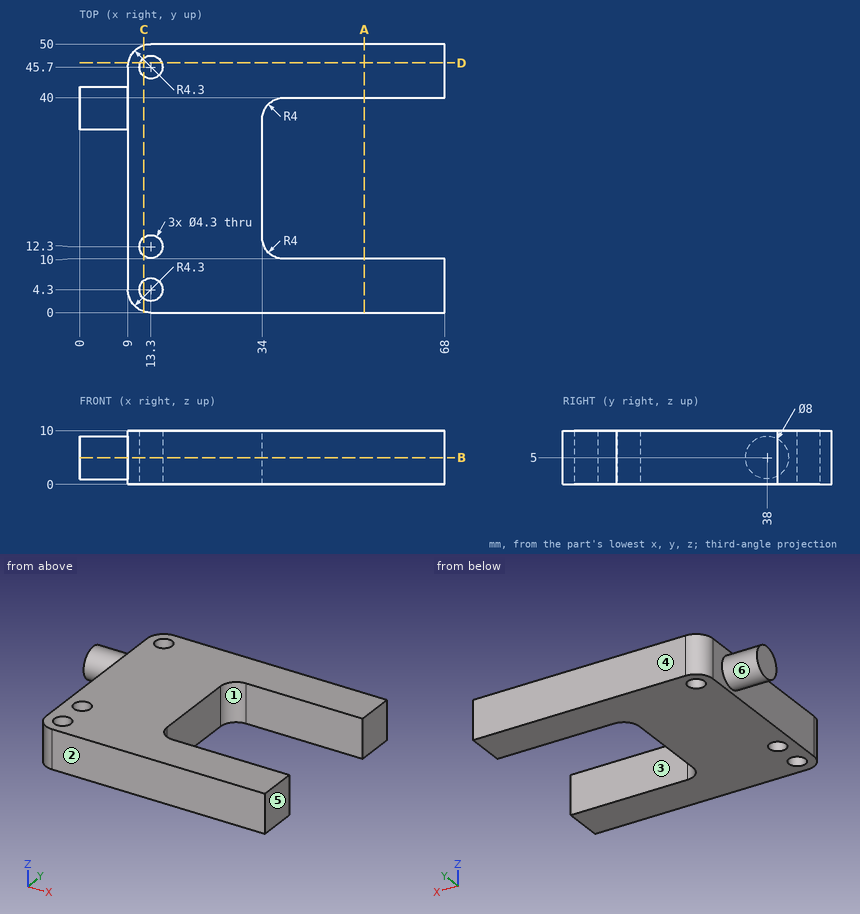
Could you check a few things on this drawing? It's one solid part, dimensions in mm from its lowest x, y, z. A direction names the side the tool comes from. Give positions to 0.01 mm unless a question says otherwise; leave off trailing zeros. Order: outer loops, then holes, each group sorted by start corner. A loop starts at its lowest first (then second) coordinate and runs counter-clockwise, first axis right, second up. Notation, with made-up numbers: (65, -18) - (69, -18) arc R34 cw to (69, 14) - close; hole circle Ø9 at (-2, -27.5). An arc over 180 degrees is marked (long way). One line per question, with ' | ' between items. Start each with the question number.
Item 1: Thinking about a two-plate mould opening in Y: for the marked faces 3, 4, 5 and 6, which applies, pulls with the +Y half, pulls with the -Y half, needs draft (parallel to the pull), parting line crosses it, or undercut?
Item 2: I need wall thicknesses on probe 1 along Y at (x, z) = (13.3, 4.75); probe 2 along Y at (x, z) = (41.5, 1.25); probe 3 along X at (y, z) = (36, 7.5). Which ranges of each line are inside material? Lowest first, please. Write a range as [from, to].
Item 3: I want a section at B-B on z = 5. Write out the boundary of the cut face in (x, y).
Item 4: I want a section at C-C on x = 12. Write out the boundary of the cut face in (y, z).
Item 5: I'm going to push flat-ended pins straight in: pin 1 Ø5 at (y, z) = (19, 5.5) entering from -X; pin 2 Ø5.5 at (x, y) = (13.3, 4.3) entering from -Z; pin 3 Ø1.5 at (y, z) = (37, 6) entering from +X; pin 4 Ø5 at (y, z) = (26, 4) entering from +X. Where does each tip first touch, or does it pass through?
Item 6: For the marked faces 1 and 2, which set-ups out of +Z, -Z, +X, -X, +Y, -Y let a thin tool reach every point of the face, with its end or its side?
Item 7: I want a section at D-D on y = 46.5. Write out the boundary of the cut face in (x, z).
Item 8: I want a section at A-A on x = 53. Write out the boundary of the cut face in (y, z), then the cut area to 3 significant figures.
Verdict:
1) face 3: undercut | face 4: pulls with the +Y half | face 5: needs draft | face 6: parting line crosses it
2) probe 1: [0, 2.15], [6.45, 10.15], [14.45, 43.55], [47.85, 50] | probe 2: [0, 10], [40, 50] | probe 3: [0, 34]
3) outline: (0, 34) - (9, 34) - (9, 4.3) arc R4.3 ccw to (13.3, 0) - (68, 0) - (68, 10) - (38, 10) arc R4 cw to (34, 14) - (34, 36) arc R4 cw to (38, 40) - (68, 40) - (68, 50) - (13.3, 50) arc R4.3 ccw to (9, 45.7) - (9, 42) - (0, 42) - close; hole circle Ø4.3 at (13.3, 4.3); hole circle Ø4.3 at (13.3, 12.3); hole circle Ø4.3 at (13.3, 45.7)
4) outline: (0.2, 0) - (2.59, 0) - (2.59, 10) - (0.2, 10) - close; (6.01, 0) - (10.59, 0) - (10.59, 10) - (6.01, 10) - close; (14.01, 0) - (43.99, 0) - (43.99, 10) - (14.01, 10) - close; (47.41, 0) - (49.8, 0) - (49.8, 10) - (47.41, 10) - close
5) pin 1: x = 9 | pin 2: z = 0 | pin 3: x = 34.4 | pin 4: x = 34
6) face 1: +Z, -Z, +X | face 2: +Z, -Z, +X, -X, -Y
7) outline: (9.08, 0) - (11.3, 0) - (11.3, 10) - (9.08, 10) - close; (15.3, 0) - (68, 0) - (68, 10) - (15.3, 10) - close
8) outline: (0, 0) - (10, 0) - (10, 10) - (0, 10) - close; (40, 0) - (50, 0) - (50, 10) - (40, 10) - close | area: 200 mm^2
